Source: CAD feature listing. Evaluate the final solid. Frame: model axes, mm. A direction names the side the tool comes from. Give positions to 0.01 mm unless a question says otherwise; leave off trailing zeros. Loops run counter-clockwise (first coordinate to the right, second up) from the corner with the lowest first, then second, coordinate; pieces in that order, holes last. Notation, with made-up numbers: M 25,-21 L 33,-21 A22 ccw 33,-4 Z; hole C 81.5,39 d10. An arc over 180 degrees is marked long. Put each result on its own line as item: value.
Autodesk Inventor part; units mm, degrees
ref_plane "YZ Plane" through (0, 0, 0) normal (1, 0, 0) x (0, 1, 0)
ref_plane "XZ Plane" through (0, 0, 0) normal (0, 1, 0) x (-1, 0, 0)
ref_plane "XY Plane" through (0, 0, 0) normal (0, 0, 1) x (1, 0, 0)
sketch "Sketch1" plane through (0, 0, 0) normal (1, 0, 0) x (0, 1, 0)
  line L0 (44.4049, 39.363) -> (-19.0951, 39.363)
  line L1 (-19.0951, 39.363) -> (-19.0951, -63.507)
  line L2 (-19.0951, -63.507) -> (44.4049, -63.507)
  line L3 (44.4049, -63.507) -> (44.4049, 39.363)
  point P0 (0, 0)
  dimension "d0" = 102.87
  dimension "d1" = 63.5
extrude "Extrusion1" add sketch "Sketch1" along normal blind 5.08
sketch "Sketch2" plane through (5.08, 0, 0) normal (1, 0, 0) x (0, 0, -1)
  line L0 (63.507, 44.4049) -> (-39.363, 44.4049)
  line L1 (-39.363, 44.4049) -> (-39.363, -19.0951)
  point P0 (0, 0)
  point P1 (-34.283, 39.3249)
  point P2 (54.617, 39.3249)
  point P3 (54.617, -8.3001)
  point P4 (-34.283, -8.3001)
  dimension "d4" = 0
  dimension "d5" = 0
  dimension "d6" = 0
  dimension "d7" = 0
  dimension "d8" = 88.9
  dimension "d9" = 5.08
  dimension "d10" = 5.08
  dimension "d11" = 47.625
hole "Hole1" at (5.08, 39.3249, 34.283) at (5.08, 39.3249, -54.617) at (5.08, -8.3001, -54.617) at (5.08, -8.3001, 34.283) direction (-1, 0, 0) diameter 5.1054 end through all
fillet "Fillet1" radius 6.35 2 edges at (2.54, 44.4049, 39.363) (2.54, 44.4049, -63.507)
sketch "Sketch7" plane through (0, -19.0951, 39.363) normal (0, 0, 1) x (1, 0, 0)
  line L0 (0, 0) -> (5.08, 0)
  line L1 (5.08, 0) -> (5.08, -5.08)
  line L2 (5.08, -5.08) -> (-40.64, -5.08)
  line L3 (-40.64, -5.08) -> (-40.64, 0)
  line L4 (-40.64, 0) -> (0, 0)
  line L5 (0, 0) -> (0, 0)
  line L6 (0, 0) -> (5.08, 0)
  line L7 (0, 57.15) -> (0, 0)
  point P0 (0, 19.0951)
  dimension "d51" = 5.08
  dimension "d52" = 5.08
  dimension "d53" = 90
  dimension "d54" = 5.08
  dimension "d55" = 45.72
  dimension "d56" = 0
  dimension "d57" = 0
extrude "Extrusion4" add sketch "Sketch7" against normal blind 102.87
sketch "Sketch8" plane through (0, -19.0951, 39.363) normal (0, 1, 0) x (1, 0, 0)
  line L0 (0, 0) -> (0, 102.87)
  line L1 (-40.64, 0) -> (0, 0)
  line L2 (-40.64, 102.87) -> (0, 102.87)
  line L3 (-40.64, 0) -> (-40.64, 102.87)
  point P0 (0, 39.363)
  point P1 (-10.16, 25.4)
  point P2 (-35.56, 25.4)
  point P3 (-35.56, 76.2)
  point P4 (-10.16, 76.2)
  dimension "d67" = 0
  dimension "d69" = 0
  dimension "d71" = 0
  dimension "d72" = 0
  dimension "d143" = 5.08
  dimension "d144" = 26.67
  dimension "d145" = 50.8
  dimension "d146" = 25.4
hole "Hole3" at (-10.16, -19.0951, 13.963) at (-35.56, -19.0951, 13.963) at (-35.56, -19.0951, -36.837) at (-10.16, -19.0951, -36.837) direction (0, -1, 0) diameter 5.1054 end through all
fillet "Fillet2" radius 6.35 2 edges at (-40.64, -21.6351, -63.507) (-40.64, -21.6351, 39.363)
sketch "Sketch9" plane through (5.08, 0, 0) normal (1, 0, 0) x (0, 0, -1)
  line L0 (57.157, 44.4049) -> (-33.013, 44.4049)
  line L1 (-39.363, 38.0549) -> (-39.363, -24.1751)
  line L2 (63.507, 38.0549) -> (63.507, -24.1751)
  point P0 (0, 0)
  point P1 (-11.423, 19.0049)
  point P2 (33.577, 19.0049)
  dimension "d82" = 0
  dimension "d83" = 45
  dimension "d84" = 25.4
  dimension "d85" = 27.94
  dimension "d86" = 29.93
hole "Hole4" at (5.08, 19.0049, 11.423) at (5.08, 19.0049, -33.577) direction (-1, 0, 0) diameter 3.048 end through all
sketch "Sketch10" plane through (0, 0, 0) normal (-1, 0, 0) x (0, 0, 1)
  line L0 (-29.767, 41.8649) -> (8.333, 41.8649)
  line L1 (8.333, 41.8649) -> (8.333, 31.7049)
  line L2 (8.333, 31.7049) -> (-29.767, 31.7049)
  line L3 (-29.767, 31.7049) -> (-29.767, 41.8649)
  line L4 (-57.157, 44.4049) -> (33.013, 44.4049)
  circle A0 centre (-33.577, 19.0049) radius 1.524
  circle A1 centre (11.423, 19.0049) radius 1.524
  point P0 (0, 0)
  dimension "d94" = 10.16
  dimension "d95" = 38.1
  dimension "d96" = 2.54
  dimension "d97" = 3.81
  dimension "d98" = 3.09
extrude "Extrusion5" add sketch "Sketch10" along normal blind 2.54 contours L0 L1 L2 L3
sketch "Sketch11" plane through (-2.54, 0, 0) normal (-1, 0, 0) x (0, 0, 1)
  line L0 (-29.767, 31.7049) -> (8.333, 31.7049)
  line L1 (-29.767, 41.8649) -> (-29.767, 31.7049)
  line L2 (8.333, 41.8649) -> (-29.767, 41.8649)
  line L3 (8.333, 31.7049) -> (8.333, 41.8649)
  point P0 (0, 0)
  point P1 (-23.417, 39.8329)
  point P2 (1.983, 39.8329)
  dimension "d101" = 0
  dimension "d102" = 25.4
  dimension "d103" = 6.35
  dimension "d104" = 8.128
hole "Hole5" at (-2.54, 39.8329, -23.417) at (-2.54, 39.8329, 1.983) direction (1, 0, 0) diameter 1.778 end through all
sketch "Sketch12" plane through (5.08, 0, 0) normal (1, 0, 0) x (0, 0, -1)
  line L0 (-39.363, -24.1751) -> (63.507, -24.1751)
  line L1 (63.507, 38.0549) -> (63.507, -24.1751)
  point P0 (0, 0)
  point P1 (31.122, 6.8129)
  point P2 (-10.4756, 6.8129)
  point P3 (-10.4756, -8.9351)
  point P4 (31.122, -8.9351)
  dimension "d112" = 41.5976
  dimension "d113" = 0
  dimension "d114" = 0
  dimension "d115" = 15.748
  dimension "d116" = 0
  dimension "d117" = 0
  dimension "d118" = 15.24
  dimension "d119" = 32.385
hole "Hole6" at (5.08, 6.8129, -31.122) at (5.08, 6.8129, 10.4756) at (5.08, -8.9351, 10.4756) at (5.08, -8.9351, -31.122) direction (-1, 0, 0) diameter 1 end through all
sketch "Sketch14" plane through (5.08, 0, 0) normal (1, 0, 0) x (0, 0, -1)
  line L0 (-8.6976, 9.3529) -> (29.344, 9.3529)
  line L1 (29.344, 9.3529) -> (29.344, 4.2729)
  line L2 (29.344, 4.2729) -> (-8.6976, 4.2729)
  line L3 (-8.6976, 4.2729) -> (-8.6976, 9.3529)
  line L4 (-8.6976, -6.3951) -> (29.344, -6.3951)
  line L5 (29.344, -6.3951) -> (29.344, -11.4751)
  line L6 (29.344, -11.4751) -> (-8.6976, -11.4751)
  line L7 (-8.6976, -11.4751) -> (-8.6976, -6.3951)
  circle A0 centre (31.122, -8.9351) radius 0.5
  circle A1 centre (31.122, 6.8129) radius 0.5
  circle A2 centre (-10.4756, 6.8129) radius 0.5
  circle A3 centre (-10.4756, -8.9351) radius 0.5
  point P0 (0, 0)
  dimension "d133" = 2.54
  dimension "d134" = 2.54
  dimension "d135" = 1.778
  dimension "d136" = 1.778
  dimension "d137" = 0
  dimension "d138" = 0
  dimension "d139" = 2.54
  dimension "d140" = 2.54
extrude "Extrusion7" cut sketch "Sketch14" against normal blind 20.725 contours L0 L1 L2 L3 | L4 L5 L6 L7
properties part number "Realsense100"
1. Contact query for flat-ended pins moving along their axis: P1, Ø10, axis at y = 7, z = 3, coming from the -X side; P2, Ø5, axis at x = -11.5, z = -47, coming from the +Y side. Output: stop coordinate, or through.
Found:
P1: x = 0
P2: y = -19.1
2. Section query A-A (x = -10.16). Output: boundary loops of the cut face in (y, z).
Found:
outline: M -24.18,-63.51 L -19.1,-63.51 L -19.1,-39.39 L -24.18,-39.39 Z; M -24.18,-34.28 L -19.1,-34.28 L -19.1,11.41 L -24.18,11.41 Z; M -24.18,16.52 L -19.1,16.52 L -19.1,39.36 L -24.18,39.36 Z
3. Access query for faces 5 (the flat face through (3, -11.475, -11)), 6 (the flat face through (1, -4, -63.507)), 7 (the flat face through (-1, 31.705, -10)), 8 (the flat face through (-1, 37, 8.333)). Directions: +Z, -Z, +X, -X, +Y, -Y. A direction counts if a zero-diameter tool reaches every point of the face in a straight line with its end or side. Return the directions, or none.
Found:
face 5: +X, -X
face 6: -Z, +X, -X, +Y, -Y
face 7: +Z, -Z, -X
face 8: +Z, -X, +Y
4. Section query C-C (z = 24). Output: boundary loops of the cut face in (x, y).
Found:
outline: M -40.64,-24.18 L 5.08,-24.18 L 5.08,44.4 L 0,44.4 L 0,-19.1 L -40.64,-19.1 Z
5. Section query B-B (z = 7). Output: boundary loops of the cut face in (x, y), plus the area to 3 significant figures.
Found:
outline: M -40.64,-24.18 L 5.08,-24.18 L 5.08,-11.48 L 0,-11.48 L 0,-19.1 L -40.64,-19.1 Z; M -2.54,31.7 L 0,31.7 L 0,9.35 L 5.08,9.35 L 5.08,44.4 L 0,44.4 L 0,41.86 L -2.54,41.86 Z; M 0,-6.4 L 5.08,-6.4 L 5.08,4.27 L 0,4.27 Z
area: 529 mm^2
6. Material intervals for line 1 (Y direction, x = 2.5, z = -3.5); line 2 (Z direction, x = -10, y = -21); line 3 (Z direction, x = -35.56, y = -23.1), sorted ascending. Write a range as from..to.
Found:
line 1: -24.18..-11.48, -6.4..4.27, 9.35..44.4
line 2: -63.51..-39.38, -34.29..11.42, 16.51..39.36
line 3: -63.38..-39.39, -34.28..11.41, 16.52..39.23
7. Section query D-D (x = -35.56). Output: boundary loops of the cut face in (y, z), plus the area to 3 significant figures.
Found:
outline: M -24.18,-63.38 L -19.1,-63.38 L -19.1,-39.39 L -24.18,-39.39 Z; M -24.18,-34.28 L -19.1,-34.28 L -19.1,11.41 L -24.18,11.41 Z; M -24.18,16.52 L -19.1,16.52 L -19.1,39.23 L -24.18,39.23 Z
area: 469 mm^2
8. Draft query along Y for faces 1 (the cylindrical face through (2.504, 41.817, 34.836)), 2 (the cylindrical face through (2.576, 42.495, -61.696)), 3 (the cylindrical face through (2.5, -10.03, -52.74)), 4 (the flat face through (-1, 37, -29.767)). Return one class per face: pulls with the +Y half, pulls with the -Y half, needs draft (parallel to the pull), parting line crosses it, or undercut.
Found:
face 1: undercut
face 2: pulls with the +Y half
face 3: undercut
face 4: needs draft
